The model under review builds one solid part; all positions refer to its coordinate system, in mm. Face numbers are marked on the shaded views. A direction names the side the tool comes from. Round coordinates to 2 decimals unless told otherwise and drop trailing zeros. Loops run counter-clockwise (first coordinate to the right, second up) from the corner with the lowest first, then second, coordinate; pieces in that order, holes last. Notation, with made-up numbers: M 10.25,-10 L 56.25,-10 A18 cw 56.25,-4 Z; hole C 3.5,48 d10. An arc over 180 degrees is marked long. One line per question, with ' | ' between items.
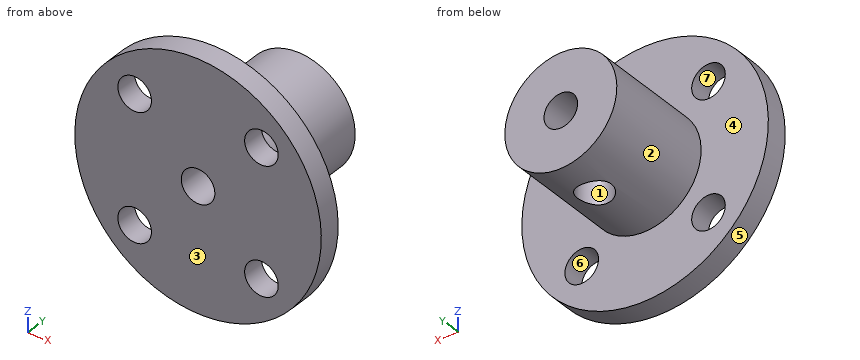
from build123d import *

# Parameters (mm, degrees)
SKETCH_1_R          = 11
SKETCH_1_R_2        = 1.5
EXTRUDE_1_DEPTH     = 2
SKETCH_2_R          = 5
SKETCH_2_R_2        = 1.5
EXTRUDE_2_DEPTH     = 10
SKETCH_3_R          = 1.5
CUT_EXTRUDE_1_DEPTH = 8


with BuildPart() as part:
    # 草图1 → 凸台-拉伸1 (new body)
    with BuildSketch(Plane(origin=(0, 0, 0), x_dir=(1, 0, 0), z_dir=(0, 1, 0))):
        with Locations(Location((0, 0, 0), (0, 0, 270))):
            Circle(SKETCH_1_R)
        with Locations(Location((0, 0, 0), (0, 0, 270))):
            Circle(SKETCH_1_R_2, mode=Mode.SUBTRACT)
        with Locations(Location((5.656854249, 5.656854249, 0), (0, 0, 270))):
            Circle(SKETCH_1_R_2, mode=Mode.SUBTRACT)
        with Locations(Location((-5.656854249, 5.656854249, 0), (0, 0, 270))):
            Circle(SKETCH_1_R_2, mode=Mode.SUBTRACT)
        with Locations(Location((-5.656854249, -5.656854249, 0), (0, 0, 270))):
            Circle(SKETCH_1_R_2, mode=Mode.SUBTRACT)
        with Locations(Location((5.656854249, -5.656854249, 0), (0, 0, 270))):
            Circle(SKETCH_1_R_2, mode=Mode.SUBTRACT)
    extrude(amount=EXTRUDE_1_DEPTH)

    # 草图2 → 凸台-拉伸2 (add)
    with BuildSketch(Plane(origin=(0, 2, 0), x_dir=(1, 0, 0), z_dir=(0, 1, 0))):
        with Locations(Location((0, 0, 0), (0, 0, 270))):
            Circle(SKETCH_2_R)
        with Locations(Location((0, 0, 0), (0, 0, 270))):
            Circle(SKETCH_2_R_2, mode=Mode.SUBTRACT)
    extrude(amount=EXTRUDE_2_DEPTH)

    # 草图3 → 切除-拉伸1 (cut)
    with BuildSketch(Plane.XY):
        with Locations((0, 8)):
            Circle(SKETCH_3_R)
    extrude(amount=-CUT_EXTRUDE_1_DEPTH, mode=Mode.SUBTRACT)


solid = part.part
1) Mouldability with a two-part tool opening along Z and no side actions: class the marked faces 4, 5, 6 and 7 as +Z half, -Z half, draft (parallel to the pull), parting line (faces both ways), or undercut.
Output values:
face 4: draft | face 5: parting line | face 6: undercut | face 7: undercut
2) Machinability: for the marked faces 1, 2 and 3, which of the approach directions +Z, -Z, +X, -X, +Y, -Y give a long, thin tool a straight path to every point of the face, cutting with its end or side? Answer none if there is none.
Output values:
face 1: -Z | face 2: +Y | face 3: +Z, -Z, +X, -X, -Y
3) Insertion check: P1, Ø2, axis at y = 2.5, z = -1.5, coming from the +X side; P2, Ø1.8, axis at x = -5.66, z = -5.66, coming from the -Y side; P3, Ø5, axis at x = -5.66, z = 5.66, coming from the +Y side; P4, Ø2.5, axis at x = 0, y = 8, coming from the +Z side. Each pin has a flat end and moves straight along its axis. Give the tip position at first contact, or say it passes through.
Output values:
P1: stops at x = 10.98 | P2: passes through | P3: stops at y = 2 | P4: stops at z = 5
4) Add section C-C on y = 5.75. State the section outline as (x, z) points, then the cut area to 3 significant figures.
Output values:
outline: C 0,0 d10; hole C 0,0 d3 | area: 71.5 mm²
5) For line 1 (X direction, y = 0.5, z = 6.75); line 2 (Y direction, x = -4, z = -4.5); line 3 (X direction, y = 7.5, z = -3.75), list the stretches that pass through material, from the lowest coordinate up.
Output values:
line 1: x = -8.69 to -6.68, -4.63 to 4.63, 6.68 to 8.69 | line 2: y = 0 to 2 | line 3: x = -3.31 to -1.41, 1.41 to 3.31
6) Add section D-D on z = -3.25. State the section outline as (x, y) points, then the cut area to 3 significant figures.
Output values:
outline: M -10.51,0 L 10.51,0 L 10.51,2 L 3.8,2 L 3.8,12 L -3.8,12 L -3.8,2 L -10.51,2 Z; hole C 0,8 d3 | area: 111 mm²
7) Add section B-B on z = 5.75. State the section outline as (x, y) points.
Output values:
outline: M -9.38,0 L -7.15,0 L -7.15,2 L -9.38,2 Z; M -4.16,0 L 4.16,0 L 4.16,2 L -4.16,2 Z; M 7.15,0 L 9.38,0 L 9.38,2 L 7.15,2 Z
8) Add section A-A on x = 0. State the section outline as (y, z) points, then the cut area to 3 significant figures.
Output values:
outline: M 0,-11 L 2,-11 L 2,-5 L 6.5,-5 L 6.5,-1.5 L 0,-1.5 Z; M 0,1.5 L 12,1.5 L 12,5 L 2,5 L 2,11 L 0,11 Z; M 9.5,-5 L 12,-5 L 12,-1.5 L 9.5,-1.5 Z | area: 97.5 mm²
